Design review of the part built by this model. Coordinates are the model's own, in mm. A direction names the side the tool comes from. Coordinates: 2 decimals unless noted, no trailing zeros. Loops run counter-clockwise (first coordinate to the right, second up) from the corner with the lowest first, then second, coordinate; pieces in that order, holes last. Notation, with made-up numbers: M 74,3 L 108,3 A31 cw 108,34 Z; hole C -36.75,-29.5 d9. An arc over 180 degrees is marked long. One line per item, written item: value.
```python
from build123d import *

# Parameters (mm, degrees)
SKETCH1_W                                  = 63
SKETCH1_H                                  = 63
SKETCH1_R                                  = 2
BOSS_EXTRUDE1_DEPTH                        = 5
SKETCH3_W                                  = 45
SKETCH3_H                                  = 45
CUT_EXTRUDE1_DEPTH                         = 5
FILLET1_R                                  = 3
SKETCH4_R                                  = 3.5
CUT_EXTRUDE2_DEPTH                         = 8
FILLET2_R                                  = 2
SKETCH5_R                                  = 5
CUT_EXTRUDE3_DEPTH                         = 2.5
MIRROR1_AT_THE_SECOND_PLANE_COPY_1_SKETC_R = 5
MIRROR1_AT_THE_SECOND_PLANE_COPY_1_DEPTH   = 2.5
FILLET3_R                                  = 2


with BuildPart() as part:
    # Sketch1 → Boss-Extrude1 (new, symmetric)
    with BuildSketch(Plane.XY):
        Rectangle(SKETCH1_W, SKETCH1_H)
        with Locations((-27.5, 27.5)):
            Circle(SKETCH1_R, mode=Mode.SUBTRACT)
        with Locations((27.5, 27.5)):
            Circle(SKETCH1_R, mode=Mode.SUBTRACT)
        with Locations((27.5, -27.5)):
            Circle(SKETCH1_R, mode=Mode.SUBTRACT)
        with Locations((-27.5, -27.5)):
            Circle(SKETCH1_R, mode=Mode.SUBTRACT)
    extrude(amount=BOSS_EXTRUDE1_DEPTH, both=True)

    # Sketch3 → Cut-Extrude1 (cut)
    with BuildSketch(Plane.XY.offset(5)):
        Rectangle(SKETCH3_W, SKETCH3_H)
    extrude(amount=-CUT_EXTRUDE1_DEPTH, mode=Mode.SUBTRACT)

    # Fillet1
    fillet1_edges = [part.edges().sort_by_distance(p)[0] for p in [
        (-31.5, 31.5, 0),
        (31.5, 31.5, 0),
        (31.5, -31.5, 0),
        (-31.5, -31.5, 0),
    ]]
    fillet(fillet1_edges, radius=FILLET1_R)

    # Sketch4 → Cut-Extrude2 (cut)
    with BuildSketch(Plane.XY.offset(5)):
        Circle(SKETCH4_R)
    extrude(amount=-CUT_EXTRUDE2_DEPTH, mode=Mode.SUBTRACT)

    # Fillet2
    fillet2_edges = [part.edges().sort_by_distance(p)[0] for p in [
        (-22.5, -22.5, 2.5),
        (-22.5, 22.5, 2.5),
        (22.5, 22.5, 2.5),
        (22.5, -22.5, 2.5),
    ]]
    fillet(fillet2_edges, radius=FILLET2_R)

    # Sketch5 → Cut-Extrude3 (cut)
    with BuildSketch(Plane(origin=(0, 0, -5), x_dir=(-1, 0, 0), z_dir=(0, 0, -1))):
        with Locations((-27.5, 27.5)):
            Circle(SKETCH5_R)
    cut_extrude3 = extrude(amount=-CUT_EXTRUDE3_DEPTH, mode=Mode.SUBTRACT)

    # Mirror1: Cut-Extrude3 across plane
    add(cut_extrude3.mirror(Plane(origin=(0, 0, 0), x_dir=(0, 0, 1), z_dir=(1, 0, 0))), mode=Mode.SUBTRACT)

    # Mirror1 at the second plane: Cut-Extrude3 across plane
    add(cut_extrude3.mirror(Plane.ZX), mode=Mode.SUBTRACT)

    # Mirror1 at the second plane copy 1 sketc → Mirror1 at the second plane copy 1 (cut)
    with BuildSketch(Plane(origin=(0, 0, -5), x_dir=(1, 0, 0), z_dir=(0, 0, -1))):
        with Locations((-27.5, 27.5)):
            Circle(MIRROR1_AT_THE_SECOND_PLANE_COPY_1_SKETC_R)
    extrude(amount=-MIRROR1_AT_THE_SECOND_PLANE_COPY_1_DEPTH, mode=Mode.SUBTRACT)

    # Fillet3
    fillet3_edges = [part.edges().sort_by_distance(p)[0] for p in [
        (24.5, 31.5, -3.75),
        (31.5, 24.5, -3.75),
        (31.5, -24.5, -3.75),
        (24.5, -31.5, -3.75),
        (-24.5, 31.5, -3.75),
        (-31.5, 24.5, -3.75),
        (-31.5, -24.5, -3.75),
        (-24.5, -31.5, -3.75),
    ]]
    fillet(fillet3_edges, radius=FILLET3_R)


solid = part.part
```
(1) To check wall thickness, follow line 1 along Y through (x, z) = (-27.5, 1.25); line 2 along Y through (x, z) = (0, -1). State the ranges of each line that lie inside material, in increasing order. Write a range as [from, to].
Reply:
line 1: y = [-31.5, -29.5], [-25.5, 25.5], [29.5, 31.5]
line 2: y = [-31.5, -3.5], [3.5, 31.5]
(2) We need section A-A on y = 27.5. State the section outline as (x, z) points.
Reply:
outline: M -31.5,-2.5 L -29.5,-2.5 L -29.5,5 L -31.5,5 Z; M -25.5,-2.5 L -22.5,-2.5 L -22.5,-5 L 22.5,-5 L 22.5,-2.5 L 25.5,-2.5 L 25.5,5 L -25.5,5 Z; M 29.5,-2.5 L 31.5,-2.5 L 31.5,5 L 29.5,5 Z
(3) Tool access review of faces 4 (the cylindrical face through (-26.577, 25.726, 1.197)), 5 (the cylindrical face through (24.02, 23.91, -3.77)), 6 (the cylindrical face through (21.9, -21.93, 2.46)): name each direction out of +Z, -Z, +X, -X, +Y, -Y from which nothing blocks a thin tool from reaching the whole face with its end or side.
Reply:
face 4: +Z, -Z
face 5: -Z
face 6: +Z
(4) Insertion check: pin 1 (5.5 mm diameter, centred on x = 0.5, y = 0, fed in from +Z); pin 2 (4.5 mm diameter, centred on x = 27.5, y = -27.5, fed in from -Z); pin 3 (13.5 mm diameter, centred on x = 8.5, y = 3.5, fed in from +Z). Each pin has a flat end and moves straight along its axis. Give the tip position at first contact, or say it passes through.
Reply:
pin 1: stops at z = -3
pin 2: stops at z = -2.5
pin 3: stops at z = 0
(5) We need section D-D on x = 18. State the section outline as (y, z) points, then the cut area to 3 significant figures.
Reply:
outline: M -31.5,-5 L 31.5,-5 L 31.5,5 L 22.5,5 L 22.5,0 L -22.5,0 L -22.5,5 L -31.5,5 Z
area: 405 mm2
(6) We need section B-B on z = 4. State the section outline as (x, y) points, then the cut area to 3 significant figures.
Reply:
outline: M -31.5,-28.5 A3 ccw -28.5,-31.5 L 28.5,-31.5 A3 ccw 31.5,-28.5 L 31.5,28.5 A3 ccw 28.5,31.5 L -28.5,31.5 A3 ccw -31.5,28.5 Z; hole C -27.5,-27.5 d4; hole C -27.5,27.5 d4; hole M -22.5,-20.5 A2 ccw -20.5,-22.5 L 20.5,-22.5 A2 ccw 22.5,-20.5 L 22.5,20.5 A2 ccw 20.5,22.5 L -20.5,22.5 A2 ccw -22.5,20.5 Z; hole C 27.5,-27.5 d4; hole C 27.5,27.5 d4
area: 1,890 mm2
(7) Mouldability with a two-part tool opening along Y and no side actions: class faces 1 (the cylindrical face through (-30.674, -22.411, -3.768)), 2 (the cylindrical face through (24.02, -23.91, -3.77)), 3 (the cylindrical face through (30.674, 22.411, -3.768)) as released by +Y, released by -Y, zero draft, split by the parting line, or undercut.
Reply:
face 1: released by -Y
face 2: undercut
face 3: released by +Y
